The listing builds one solid part. Answer for the finished solid, in the listing's coordinates (mm). A direction names the side the tool comes from. Coordinates: 2 decimals unless noted, no trailing zeros. Write each loop counter-clockwise with the first axis right and the second up, starting at its lowest first coordinate (ties: lowest second). Pieces come first, ordered by that corner, then holes.
(1) The part is cut by section A-A on x = 10.5. Determine the outline of the cut face in (y, z).
(2) Given P1, Ø0.9, axis at x = 6, z = 0.5, coming from the +Y side; P2, Ø2.5, axis at y = -12, z = -12, coming from the -X side; P3, Ø3, axis at x = -5, z = -1.5, coming from the -Y side; P4, Ø0.5, axis at x = -0.5, y = 10.5, coming from the -Z side, each flat-ended and moving along its own axis, determine where each tip first touches the part or whether it passes through.
(3) The part is cut by section D-D on y = -12. Give the number of separate pieces and of enclosed holes in the cut face, plus the area to 3 significant figures.
(4) Straight lines are drawn through the part: line 1 (Y direction, x = -12, z = 12); line 2 (X direction, y = 16.5, z = -4); line 3 (Y direction, x = 0, z = -9). For each, find the intervals that lie inside material, in ascending order.
(5) For a pull along X with two mould halves and no side action, classify faces 4 (the flat face through (0.5, -12.51, 10.49)), 5 (the flat face through (6.479, -19.836, 2.358)), 6 (the flat face through (3.544, 18, -3)) as +X half, -X half, draft (parallel to the pull), parting line (faces both ways), or undercut.
(6) Which of the six approach directions +Z, -Z, +X, -X, +Y, -Y give full straight-line access (tool end or side, diameter ignored) to faces 1 (the flat face through (0, -12, -12)), 2 (the flat face through (5, 17, -1)), 3 (the flat face through (8, -16, -2))?
(7) The part is cut by section B-B on y = 6.5. Determine the outline of the cut face in (x, z).
from build123d import *

# Parameters (mm, degrees)
F0_W      = 2
F0_H      = 5
F5_DEPTH  = 15
F6_DEPTH  = 15
F7_DEPTH  = 16
F2_R      = 1.43
F8_DEPTH  = 25
F9_DEPTH  = 25
F3_R      = 1.5
F10_DEPTH = 8
F11_START = 5
F11_DEPTH = 20
F4_W      = 7
F4_H      = 12
F12_DEPTH = 20
F14_START = 10
F13_W     = 2
F13_H     = 30
F14_DEPTH = 1
F15_R     = 10
F16_DEPTH = 25
F17_SIZE  = 0.9999


# Not quite as in the source:
# - a fillet or chamfer is up to 0.001 mm smaller than in the source, because OpenCascade refuses the exact size


with BuildPart() as f5:
    # F0 (on Front) → F5 (new body, symmetric)
    with BuildSketch(Plane.XZ):
        Polygon((-11, 15), (-15, 15), (-15, -15), (10, -15), (10, 10), (-7, 10), align=None)
        Polygon((10, 10), (10, -15), (15, -5.5), (15, 0.5), align=None)
        with Locations((12.5, -2.5)):
            Rectangle(F0_W, F0_H, mode=Mode.SUBTRACT)
    extrude(amount=F5_DEPTH, both=True)

    # F1 (on Top) → F6 (cut, symmetric)
    with BuildSketch(Plane.XY):
        with BuildLine():
            Line((16, 10), (4.582575695, 10))
            ThreePointArc((4.582575695, 10), (-11, 0), (4.582575695, -10))
            Line((4.582575695, -10), (16, -10))
            Line((16, -10), (16, 10))
        make_face()
    extrude(amount=F6_DEPTH, both=True, mode=Mode.SUBTRACT)

    # F2 (on Right) → F7 (cut)
    with BuildSketch(Plane.YZ):
        with BuildLine():
            Line((9.0691785736, 10), (-9.0691785736, 10))
            ThreePointArc((-9.0691785736, 10), (0, -13.5), (9.0691785736, 10))
        make_face()
    extrude(amount=-F7_DEPTH, mode=Mode.SUBTRACT)

    # F2 (on Right) → F8 (cut)
    with BuildSketch(Plane.YZ):
        with Locations((12, 12)):
            Circle(F2_R)
        with Locations((-12, 12)):
            Circle(F2_R)
    extrude(amount=-F8_DEPTH, mode=Mode.SUBTRACT)

    # F2 (on Right) → F9 (cut)
    with BuildSketch(Plane.YZ):
        with Locations((12, -12)):
            Circle(F2_R)
        with Locations((-12, -12)):
            Circle(F2_R)
    extrude(amount=-F9_DEPTH, mode=Mode.SUBTRACT)

    # F3 (on Right) → F10 (join, symmetric)
    with BuildSketch(Plane.YZ):
        with BuildLine():
            Line((15, -14.5), (21.9673867507, -3.2620052331))
            ThreePointArc((21.9673867507, -3.2620052331), (22.6917908233, -0.1175906407), (21.3446249631, 2.8145158605))
            Line((21.3446249631, 2.8145158605), (15, 9.5))
            Line((15, 9.5), (15, -14.5))
        make_face()
        Polygon((18.5, 3.129238459), (21.21, 1.5646192295), (21.21, -1.5646192295), (18.5, -3.129238459), (15.79, -1.5646192295), (15.79, 1.5646192295), align=None, mode=Mode.SUBTRACT)
        Polygon((21.21, -1.5646192295), (21.21, 1.5646192295), (18.5, 3.129238459), (15.79, 1.5646192295), (15.79, -1.5646192295), (18.5, -3.129238459), align=None)
        with Locations((18.5, 0)):
            Circle(F3_R, mode=Mode.SUBTRACT)
        with BuildLine():
            Line((-15, 9.5), (-21.3446249631, 2.8145158605))
            ThreePointArc((-21.3446249631, 2.8145158605), (-22.6917908233, -0.1175906407), (-21.9673867507, -3.2620052331))
            Line((-21.9673867507, -3.2620052331), (-15, -14.5))
            Line((-15, -14.5), (-15, 9.5))
        make_face()
        Polygon((-21.21, 1.5646192295), (-18.5, 3.129238459), (-15.79, 1.5646192295), (-15.79, -1.5646192295), (-18.5, -3.129238459), (-21.21, -1.5646192295), align=None, mode=Mode.SUBTRACT)
        Polygon((-15.79, 1.5646192295), (-18.5, 3.129238459), (-21.21, 1.5646192295), (-21.21, -1.5646192295), (-18.5, -3.129238459), (-15.79, -1.5646192295), align=None)
        with Locations((-18.5, 0)):
            Circle(F3_R, mode=Mode.SUBTRACT)
    extrude(amount=F10_DEPTH, both=True)

    # F3 (on Right) → F11 (cut)
    with BuildSketch(Plane.YZ.offset(F11_START)):
        Polygon((21.21, -1.5646192295), (21.21, 1.5646192295), (18.5, 3.129238459), (15.79, 1.5646192295), (15.79, -1.5646192295), (18.5, -3.129238459), align=None)
        with Locations((18.5, 0)):
            Circle(F3_R, mode=Mode.SUBTRACT)
        with Locations((18.5, 0)):
            Circle(F3_R)
        Polygon((-15.79, 1.5646192295), (-18.5, 3.129238459), (-21.21, 1.5646192295), (-21.21, -1.5646192295), (-18.5, -3.129238459), (-15.79, -1.5646192295), align=None)
        with Locations((-18.5, 0)):
            Circle(F3_R, mode=Mode.SUBTRACT)
        with Locations((-18.5, 0)):
            Circle(F3_R)
    extrude(amount=F11_DEPTH, mode=Mode.SUBTRACT)

    # F4 (on Top) → F12 (cut, symmetric)
    with BuildSketch(Plane.XY):
        with Locations((0.0437486451, 21)):
            Rectangle(F4_W, F4_H)
        with Locations((0.0437486451, -21)):
            Rectangle(F4_W, F4_H)
    extrude(amount=F12_DEPTH, both=True, mode=Mode.SUBTRACT)

    # F13 (on Top) → F14 (join)
    with BuildSketch(Plane.XY.offset(F14_START)):
        with Locations((-0.0117724412, 0)):
            Rectangle(F13_W, F13_H)
    extrude(amount=F14_DEPTH)

    # F15 (on Top) → F16 (cut)
    with BuildSketch(Plane.XY):
        Circle(F15_R)
    extrude(amount=F16_DEPTH, mode=Mode.SUBTRACT)

    # F17 (size 1 in the source; OpenCascade refuses exactly that, so slightly less here)
    f17_edges = [f5.edges().sort_by_distance(p)[0] for p in [
        (0.988228, 12.475525, 11),
        (-1.011772, 12.474342, 11),
        (-0.011772, 15, 11),
        (0.988228, -12.475525, 11),
        (-0.011772, -15, 11),
        (-1.011772, -12.474342, 11),
    ]]
    chamfer(f17_edges, length=F17_SIZE)


solid = f5.part
Model answer:
1. outline: (-15, -14.05) - (-10, -14.05) - (-10, 9.05) - (-15, 9.05) - close; (10, -14.05) - (15, -14.05) - (15, 9.05) - (10, 9.05) - close
2. P1: stops at y = 22.67
2. P2: stops at x = 0
2. P3: stops at y = -22.72
2. P4: stops at z = 10
3. separate pieces: 2
3. enclosed holes: 1
3. area: 477 mm2
4. line 1: y = -15 to -13.43, -10.57 to 10.57, 13.43 to 15
4. line 2: x = -8 to -3.46, 3.54 to 8
4. line 3: y = -15 to -11, 11 to 15
5. face 4: +X half
5. face 5: draft
5. face 6: undercut
6. face 1: -X
6. face 2: +X
6. face 3: +Z, -Z, +X, -Y
7. outline: (-15, -15) - (-8.87, -15) - (-8.87, -11.83) - (-15, -11.83) - close; (-15, 10) - (-8.87, 10) - (-8.87, 12.34) - (-11, 15) - (-15, 15) - close
